```python
from build123d import *

# Parameters (mm, degrees)
SKETCH_1_W                   = 48
SKETCH_1_H                   = 37
EXTRUDE_1_DEPTH              = 8
SKETCH_2_W                   = 20
SKETCH_2_H                   = 22
CUT_EXTRUDE_1_DEPTH          = 32.340867888
FILLET_1_R                   = 10
SKETCH_3_W                   = 8
SKETCH_3_H                   = 6
EXTRUDE_2_DEPTH              = 1
SKETCH_4_R                   = 2
CUT_EXTRUDE_2_DEPTH          = 32.610915836
HOLE_WIZARD_M4_1_D           = 4.3
HOLE_WIZARD_M4_1_CBORE_D     = 8
HOLE_WIZARD_M4_1_CBORE_DEPTH = 4.4
SKETCH_7_W                   = 8
SKETCH_7_H                   = 8
CUT_EXTRUDE_3_DEPTH          = 5
CHAMFER_1_SIZE               = 5
FILLET_2_R                   = 3


with BuildPart() as part:
    # 草图1 → 凸台-拉伸1 (new body)
    with BuildSketch(Plane(origin=(0, 0, 0), x_dir=(1, 0, 0), z_dir=(0, 1, 0))):
        Rectangle(SKETCH_1_W, SKETCH_1_H)
    extrude(amount=EXTRUDE_1_DEPTH)

    # 草图2 → 切除-拉伸1 (cut, through all)
    with BuildSketch(Plane(origin=(0, 8, 0), x_dir=(1, 0, 0), z_dir=(0, 1, 0))):
        with Locations((-14, -7.5)):
            Rectangle(SKETCH_2_W, SKETCH_2_H)
        with Locations((14, -7.5)):
            Rectangle(SKETCH_2_W, SKETCH_2_H)
    extrude(amount=-CUT_EXTRUDE_1_DEPTH, mode=Mode.SUBTRACT)

    # 圆角1
    fillet_1_edges = [part.edges().sort_by_distance(p)[0] for p in [
        (-4, 4, -3.5),
        (4, 4, -3.5),
    ]]
    fillet(fillet_1_edges, radius=FILLET_1_R)

    # 草图3 → 凸台-拉伸2 (add)
    with BuildSketch(Plane.XZ):
        with Locations((0, 15.5)):
            Rectangle(SKETCH_3_W, SKETCH_3_H)
    extrude(amount=EXTRUDE_2_DEPTH)

    # 草图4 → 切除-拉伸2 (cut, through all)
    with BuildSketch(Plane(origin=(0, 8, 0), x_dir=(1, 0, 0), z_dir=(0, 1, 0))):
        with Locations(Location((0, -15.5, 0), (0, 0, 270))):
            Circle(SKETCH_4_R)
    extrude(amount=-CUT_EXTRUDE_2_DEPTH, mode=Mode.SUBTRACT)

    # M4 六角凹头螺钉的柱形沉头孔1 (through all)
    with Locations(Plane(origin=(17.5, 0, -11), x_dir=(0, 0, -1), z_dir=(0, -1, 0))):
        with Locations((0, 0), (0, -35)):
            CounterBoreHole(HOLE_WIZARD_M4_1_D / 2, HOLE_WIZARD_M4_1_CBORE_D / 2, HOLE_WIZARD_M4_1_CBORE_DEPTH)

    # 草图7 → 切除-拉伸3 (cut)
    with BuildSketch(Plane(origin=(0, 8, 0), x_dir=(1, 0, 0), z_dir=(0, 1, 0))):
        with Locations((0, -14.5)):
            Rectangle(SKETCH_7_W, SKETCH_7_H)
    extrude(amount=-CUT_EXTRUDE_3_DEPTH, mode=Mode.SUBTRACT)

    # 倒角1
    chamfer_1_edges = [part.edges().sort_by_distance(p)[0] for p in [
        (0, 8, 10.5),
    ]]
    chamfer(chamfer_1_edges, length=CHAMFER_1_SIZE - 0.0001)  # a hair under: the kernel refuses the full size

    # 圆角2
    fillet_2_edges = [part.edges().sort_by_distance(p)[0] for p in [
        (-4, 1, 18.5),
        (4, 1, 18.5),
    ]]
    fillet(fillet_2_edges, radius=FILLET_2_R)


solid = part.part
```
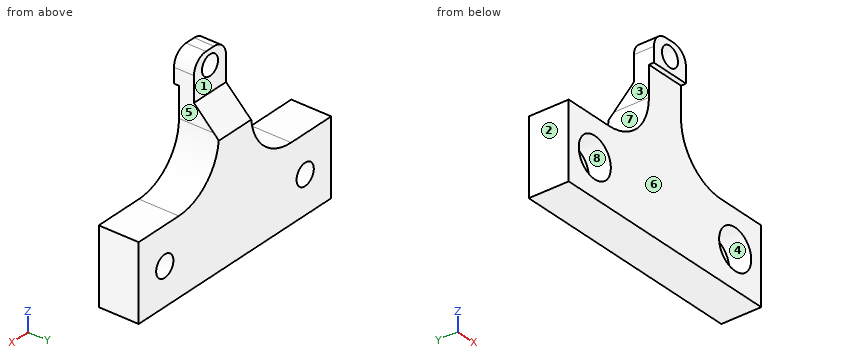
Geometry: final body of the model. Coordinates: model frame, mm. Face numbers are marked on the shaded views. A direction names the side the tool comes from. Coordinates: 2 decimals unless noted, no trailing zeros. Write each loop counter-clockwise with the first axis right and the second up, starting at its lowest first coordinate (ties: lowest second). Pieces come first, ordered by that corner, then holes. Notation, with made-up numbers: M 41,18 L 46,18 A24 ccw 46,40 Z; hole C 65.25,76.5 d4. An arc over 180 degrees is marked long. Answer as CSV lines item,"result". Start each with the question number.
Q1. Cut plane A-A on z = -11. Return the cut outline in (x, y).
Q2. Reachability of the marked faces 1, 2, 3, 4 and 5 from +Z, -Z, +X, -X, +Y, -Y: full face, straight path, thin tool, end or side. Return the list, or none.
Q3. Mould query, pull axis Z, two halves, no side actions, for the marked faces 6, 7 and 8. Classes: released by +Z, released by -Z, zero draft, split by the parting line, or undercut.
Q4. Line query: line 1 (X direction, y = 2.4, z = -11); line 2 (Z direction, x = 17, y = 4.5); line 3 (Z direction, x = -19, y = 5). Output: solid intervals per line, ascending. Write a range as from..to.
Q5. Pin query (flat end, axial travel): P1, Ø4, axis at x = 18, y = 3, coming from the +Z side; P2, Ø5, axis at y = 4, z = 2, coming from the +X side; P3, Ø2.5, axis at y = 2, z = 9.5, coming from the -X side. Return the tip coordinate at first contact, or that it passes through.
Q6. Cut plane B-B on x = 17.5. Return the cut outline in (y, z), then the cut area to 3 significant figures.
Q7. Cut plane C-C on y = 5. Return the cut outline in (x, z), then the cut area to 3 significant figures.
Findings below:
1,outline,"M -24,0 L -21.5,0 L -21.5,4.4 L -19.65,4.4 L -19.65,8 L -24,8 Z; M -15.35,4.4 L -13.5,4.4 L -13.5,0 L 13.5,0 L 13.5,4.4 L 15.35,4.4 L 15.35,8 L -15.35,8 Z; M 19.65,4.4 L 21.5,4.4 L 21.5,0 L 24,0 L 24,8 L 19.65,8 Z"
2,face 1,"+Z, +X, -X, +Y"
2,face 2,"+Z, -Z, -X, +Y, -Y"
2,face 3,"+Z, -X, +Y, -Y"
2,face 4,"-Y"
2,face 5,"+Z, +X, +Y, -Y"
3,face 6,"zero draft"
3,face 7,"released by +Z"
3,face 8,"undercut"
4,line 1,"x = -24..-21.5, -13.5..13.5, 21.5..24"
4,line 2,"z = -18.5..-13.09, -8.91..-3.5"
4,line 3,"z = -18.5..-12.54, -9.46..-3.5"
5,P1,"stops at z = -3.5"
5,P2,"stops at x = 6.86"
5,P3,"stops at x = -4"
6,outline,"M 0,-18.5 L 8,-18.5 L 8,-13.15 L 4.4,-13.15 L 4.4,-15 L 0,-15 Z; M 0,-7 L 4.4,-7 L 4.4,-8.85 L 8,-8.85 L 8,-3.5 L 0,-3.5 Z"
6,area,"69.3 mm2"
7,outline,"M -24,-18.5 L 24,-18.5 L 24,-3.5 L 14,-3.5 A10 cw 4,6.5 L 4,8.5 L -4,8.5 L -4,6.5 A10 cw -14,-3.5 L -24,-3.5 Z; hole C -17.5,-11 d4.3; hole C 17.5,-11 d4.3"
7,area,"830 mm2"
